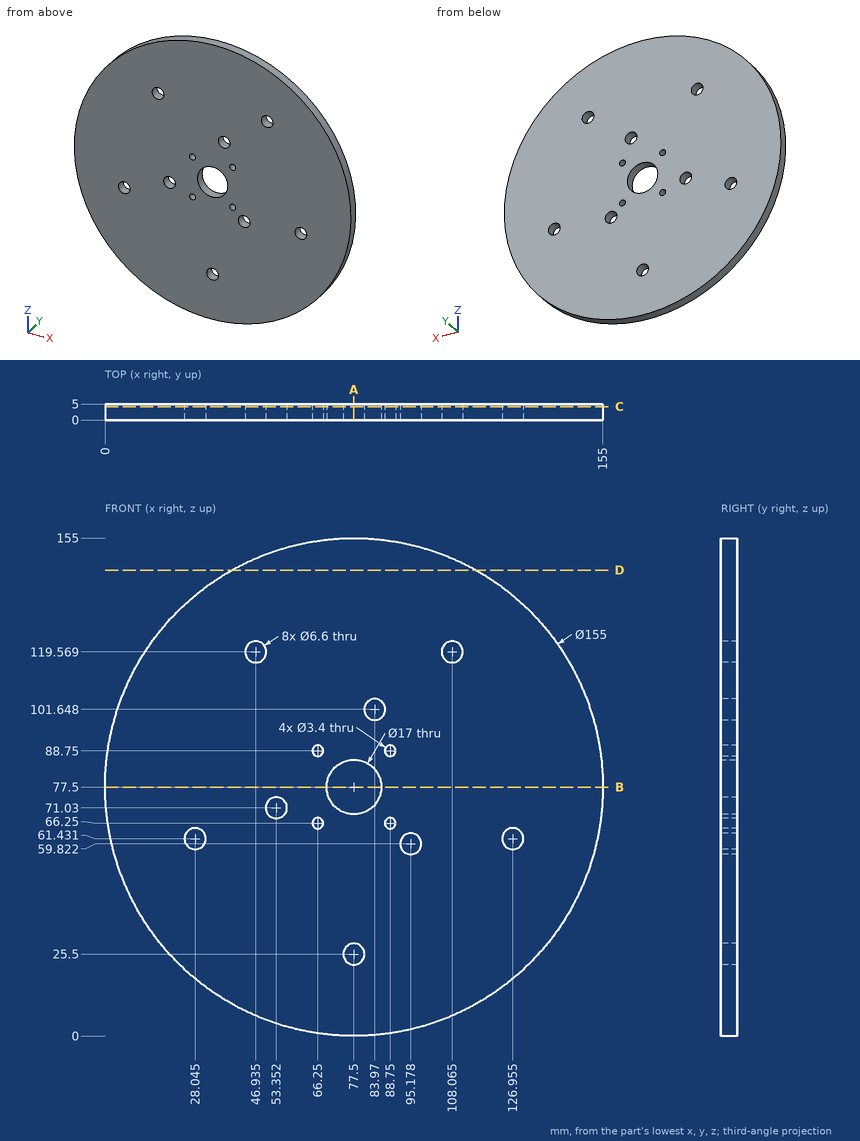
For this review, use the dimensioned drawing (mm, ordinates from the lowest corner) and the shaded views. Give positions to 0.01 mm unless a question says otherwise; leave off trailing zeros. Loops run counter-clockwise (first coordinate to the right, second up) from the corner with the lowest first, then second, coordinate; pieces in that order, holes last.
Item 1: For line 1 along Z through (x, y) = (66.25, 2.25); line 2 along X through (y, z) = (4, 119) (1 decimal); line 3 along X through (y, z) = (1.2, 62) (1 decimal), list the stretches that pass through material, from the lowest coordinate up.
Item 2: Take a section at C-C, the plane y = 4.15. Give the number of separate pieces and of enclosed holes in the cut face, and give its area (3 significant figures).
Item 3: Take a section at D-D, the plane z = 145. State the section outline as (x, y) points, and give its area (3 significant figures).
Item 4: Take a section at A-A, the plane x = 77.5. State the section outline as (y, z) points, and give its area (3 significant figures).
Item 5: Take a section at B-B, the plane z = 77.5. State the section outline as (x, y) points.
Item 6: Insertion check: pin 1 (1 mm diameter, centred on x = 33.5, y = 3, fed in from +Z). The pin has a flat end and moves straight along its axis. Give the tip position at first contact, or say it passes through.
Calculated:
1. line 1: z = 0.82 to 64.55, 67.95 to 87.05, 90.45 to 154.18
1. line 2: x = 12 to 43.7, 50.2 to 104.8, 111.3 to 143
1. line 3: x = 1.6 to 24.8, 31.3 to 92.7, 97.7 to 123.7, 130.2 to 153.4
2. separate pieces: 1
2. enclosed holes: 13
2. area: 18,300 mm2
3. outline: (39.42, 0) - (115.58, 0) - (115.58, 5) - (39.42, 5) - close
3. area: 381 mm2
4. outline: (0, 0) - (5, 0) - (5, 22.2) - (0, 22.2) - close; (0, 28.8) - (5, 28.8) - (5, 69) - (0, 69) - close; (0, 86) - (5, 86) - (5, 155) - (0, 155) - close
4. area: 657 mm2
5. outline: (0, 0) - (69, 0) - (69, 5) - (0, 5) - close; (86, 0) - (155, 0) - (155, 5) - (86, 5) - close
6. pin 1: stops at z = 141.64
